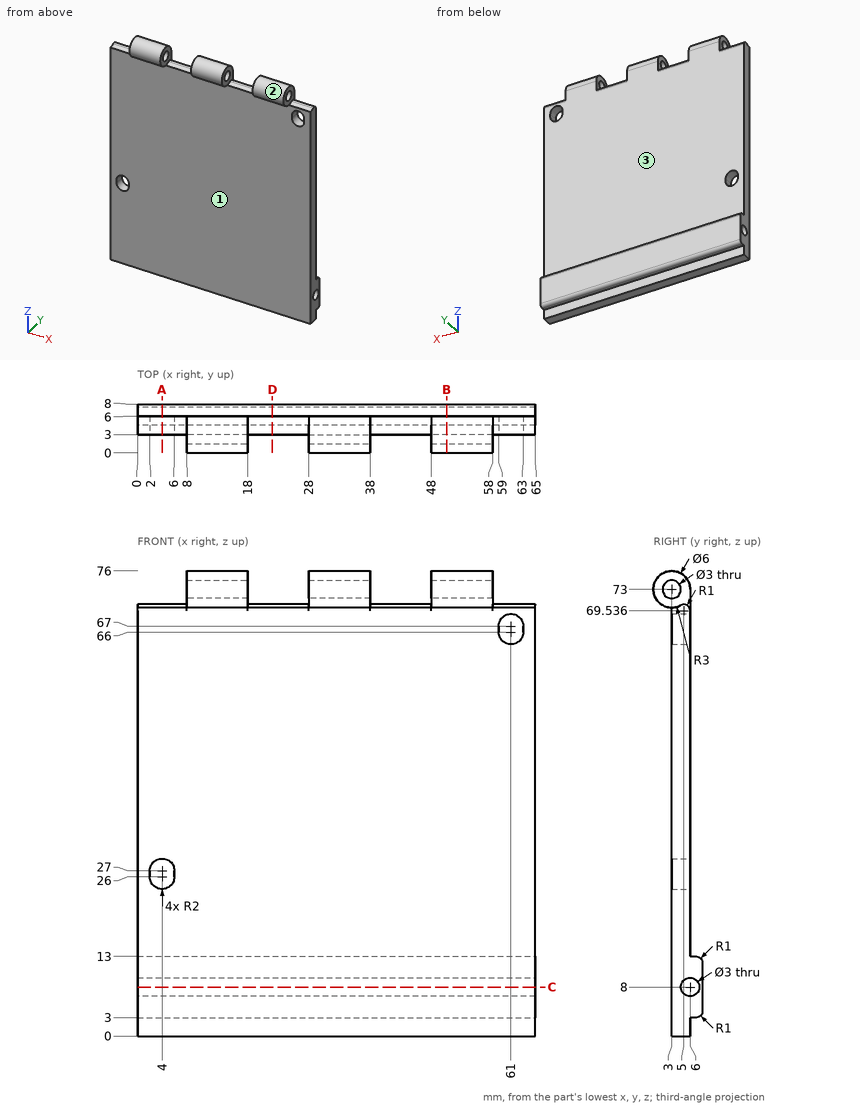
Input: dimensioned drawing with shaded views. Units: mm. Origin: part minimum x, y, z. A direction names the side the tool comes from. Round coordinates to 2 decimals unless told otherwise and drop trailing zeros. Order: outer loops, then holes, each group sorted by start corner. A loop starts at its lowest first (then second) coordinate and runs counter-clockwise, first axis right, second up. Notation, with made-up numbers: (71, -27) -> (108, -27) arc R21 ccw to (108, -5) -> close; hole circle Ø4 at (74, 41). An arc over 180 degrees is marked (long way). Put each result on its own line as item: value. Start each with the question number.
Q1. Section C-C on z = 8. Return the cut outline in (x, y), and give its area (3 significant figures).
Q2. Reachability of the marked faces 1, 2 and 3 from +Z, -Z, +X, -X, +Y, -Y: full face, straight path, thin tool, end or side. Return the list, or none.
Q3. Section A-A on x = 4. Return the cut outline in (y, z).
Q4. Section B-B on x = 50.5. Return the cut outline in (y, z), and give its area (3 significant figures).
Q5. Line query: probe 1 along Y at (x, z) = (36, 73); probe 2 along Y at (x, z) = (30.5, 32); probe 3 along Y at (x, z) = (32, 7.5). Output: solid intervals per line, ascending.
Q6. First-contact query: pin 1 (5 mm diameter, centred on x = 18.5, z = 10, fed in from -Y); pin 2 (0.8 mm diameter, centred on x = 16.5, y = 6.5, fed in from +Z); pin 3 (1.8 mm diameter, centred on y = 2, z = 72, fed in from -X); pin 4 (1.8 mm diameter, centred on y = 3, z = 72.5, fed in from -X). Flat tips, straight axial feed; report the tip coordinate or a pass-through.
Q7. Section D-D on x = 22. Return the cut outline in (y, z), and give its area (3 significant figures).
Ans:
1. outline: (0, 3) -> (65, 3) -> (65, 4.5) -> (0, 4.5) -> close; (0, 7.5) -> (65, 7.5) -> (65, 8) -> (0, 8) -> close
1. area: 130 mm2
2. face 1: -Z, +X, -X, -Y
2. face 2: +X, -X
2. face 3: +Z, +X, -X, +Y
3. outline: (3, 0) -> (6, 0) -> (6, 3) -> (7, 3) arc R1 ccw to (8, 4) -> (8, 12) arc R1 ccw to (7, 13) -> (6, 13) -> (6, 24) -> (3, 24) -> close; (3, 29) -> (6, 29) -> (6, 69.54) arc R1 ccw to (4.5, 70.4) arc R3 cw to (3, 70) -> close; hole circle Ø3 at (6, 8)
4. outline: (3, 0) -> (6, 0) -> (6, 3) -> (7, 3) arc R1 ccw to (8, 4) -> (8, 12) arc R1 ccw to (7, 13) -> (6, 13) -> (6, 73) arc R3 ccw (long way) to (3, 70) -> close; hole circle Ø3 at (3, 73); hole circle Ø3 at (6, 8)
4. area: 246 mm2
5. probe 1: y = 0 to 1.5, 4.5 to 6
5. probe 2: y = 3 to 6
5. probe 3: y = 3 to 4.59, 7.41 to 8
6. pin 1: stops at y = 3
6. pin 2: stops at z = 13
6. pin 3: stops at x = 8
6. pin 4: passes through
7. outline: (3, 0) -> (6, 0) -> (6, 3) -> (7, 3) arc R1 ccw to (8, 4) -> (8, 12) arc R1 ccw to (7, 13) -> (6, 13) -> (6, 69.54) arc R1 ccw to (4.5, 70.4) arc R3 cw to (3, 70) -> close; hole circle Ø3 at (6, 8)
7. area: 223 mm2
